from build123d import *

# Parameters (mm, degrees)
BOSS_EXTRUDE1_DEPTH = 12
SKETCH2_R           = 2.5
CUT_EXTRUDE2_DEPTH  = 15
SKETCH3_R           = 2.5
CUT_EXTRUDE4_DEPTH  = 15


with BuildPart() as part:
    # Sketch1 → Boss-Extrude1 (new body)
    with BuildSketch(Plane.XY):
        Polygon((0, 0), (150, 0), (150, 15), (15, 150), (0, 150), align=None)
    extrude(amount=BOSS_EXTRUDE1_DEPTH)

    # Sketch2 → Cut-Extrude2 (cut)
    with BuildSketch(Plane(origin=(0, 0, 0), x_dir=(1, 0, 0), z_dir=(0, 1, 0))):
        with Locations(Location((33, -6, 0), (0, 0, 270))):
            Circle(SKETCH2_R)
        with Locations(Location((113, -6, 0), (0, 0, 270))):
            Circle(SKETCH2_R)
    extrude(amount=CUT_EXTRUDE2_DEPTH, mode=Mode.SUBTRACT)

    # Sketch3 → Cut-Extrude4 (cut)
    with BuildSketch(Plane(origin=(0, 0, 0), x_dir=(0, 0, -1), z_dir=(1, 0, 0))):
        with Locations((-6, 50)):
            Circle(SKETCH3_R)
        with Locations((-6, 120)):
            Circle(SKETCH3_R)
    extrude(amount=CUT_EXTRUDE4_DEPTH, mode=Mode.SUBTRACT)


solid = part.part
Source: CAD feature listing. Evaluate the final solid. Frame: model axes, mm. A direction names the side the tool comes from. Coordinates: 2 decimals unless noted, no trailing zeros. Loops run counter-clockwise (first coordinate to the right, second up) from the corner with the lowest first, then second, coordinate; pieces in that order, holes last. Notation, with made-up numbers: (24.5, -25) - (48.5, -25) arc R10 ccw to (48.5, -16) - close; hole circle Ø7 at (46, 35). An arc over 180 degrees is marked (long way). Return JSON: item names as keys, results as strings.
Q1. Contact query for flat-ended pins moving along their axis: P1, Ø4, axis at x = 33, z = 6, coming from the +Y side; P2, Ø4, axis at x = 113, z = 6, coming from the +Y side; P3, Ø1.5, axis at y = 105.5, z = 5, coming from the +X side. Output: stop coordinate, or through.
Results:
{"P1": "y = 134", "P2": "y = 54", "P3": "x = 60.25"}
Q2. Mould query, pull axis Y, two halves, no side actions, for faces 4 (the flat face through (8, 150, 6)), 5 (the flat face through (15, 50, 6)), 6 (the flat face through (57, 59, 0)), 7 (the cylindrical face through (7.395, 50.751, 3.615)). Classes: released by +Y, released by -Y, zero draft, split by the parting line, or undercut.
Results:
{"face 4": "released by +Y", "face 5": "undercut", "face 6": "zero draft", "face 7": "undercut"}
Q3. Section B-B, the plane x = 113. Return loops of the section in (y, z), plus the area to 3 significant figures.
Results:
{"outline": "(0, 0) - (52, 0) - (52, 12) - (0, 12) - (0, 8.5) - (15, 8.5) - (15, 3.5) - (0, 3.5) - close", "area": "549 mm2"}
Q4. Section C-C, the plane y = 120. Return loops of the section in (x, z).
Results:
{"outline": "(0, 0) - (45, 0) - (45, 12) - (0, 12) - (0, 8.5) - (15, 8.5) - (15, 3.5) - (0, 3.5) - close"}
Q5. Section D-D, the plane y = 28. Return loops of the section in (x, z).
Results:
{"outline": "(0, 0) - (137, 0) - (137, 12) - (0, 12) - close"}
Q6. Material intervals for line 1 along Y through (x, z) = (3, 6); line 2 along X through (y, z) = (6, 6.5); line 3 along X through (y, z) = (7.5, 5), sorted ascending.
Results:
{"line 1": "0 to 47.5, 52.5 to 117.5, 122.5 to 150", "line 2": "0 to 30.55, 35.45 to 110.55, 115.45 to 150", "line 3": "0 to 30.71, 35.29 to 110.71, 115.29 to 150"}
Q7. Section A-A, the plane z = 6. Return loops of the section in (x, y), plus the area to 3 significant figures.
Results:
{"outline": "(0, 0) - (30.5, 0) - (30.5, 15) - (35.5, 15) - (35.5, 0) - (110.5, 0) - (110.5, 15) - (115.5, 15) - (115.5, 0) - (150, 0) - (150, 15) - (15, 150) - (0, 150) - (0, 122.5) - (15, 122.5) - (15, 117.5) - (0, 117.5) - (0, 52.5) - (15, 52.5) - (15, 47.5) - (0, 47.5) - close", "area": "13,100 mm2"}
Q8. Access query for faces 1 (the cylindrical face through (35.11, 7.4, 7.34)), 2 (the flat face through (15, 120, 6)), 3 (the flat face through (74, 0, 6)). Directions: +Z, -Z, +X, -X, +Y, -Y. A direction counts if a zero-diameter tool reaches every point of the face in a straight line with its end or side. Return the directions, or none.
Results:
{"face 1": "-Y", "face 2": "-X", "face 3": "+Z, -Z, +X, -X, -Y"}
